Geometry: see drawing. Coordinates: mm, zero at the bounding-box minimum. Give positions to 0.01 mm unless a question says otherwise; leave off trailing zeros. Write each loop counter-clockwise with the first axis right and the second up, starting at its lowest first coordinate (ties: lowest second). Pieces come first, ordered by that corner, then holes. Notation, with made-up numbers: (64, 8.5) - (101, 8.5) arc R20 cw to (101, 21.5) - close; hole circle Ø11 at (26.25, 71). An arc over 180 degrees is marked (long way). Return JSON: item names as keys, results as strings.
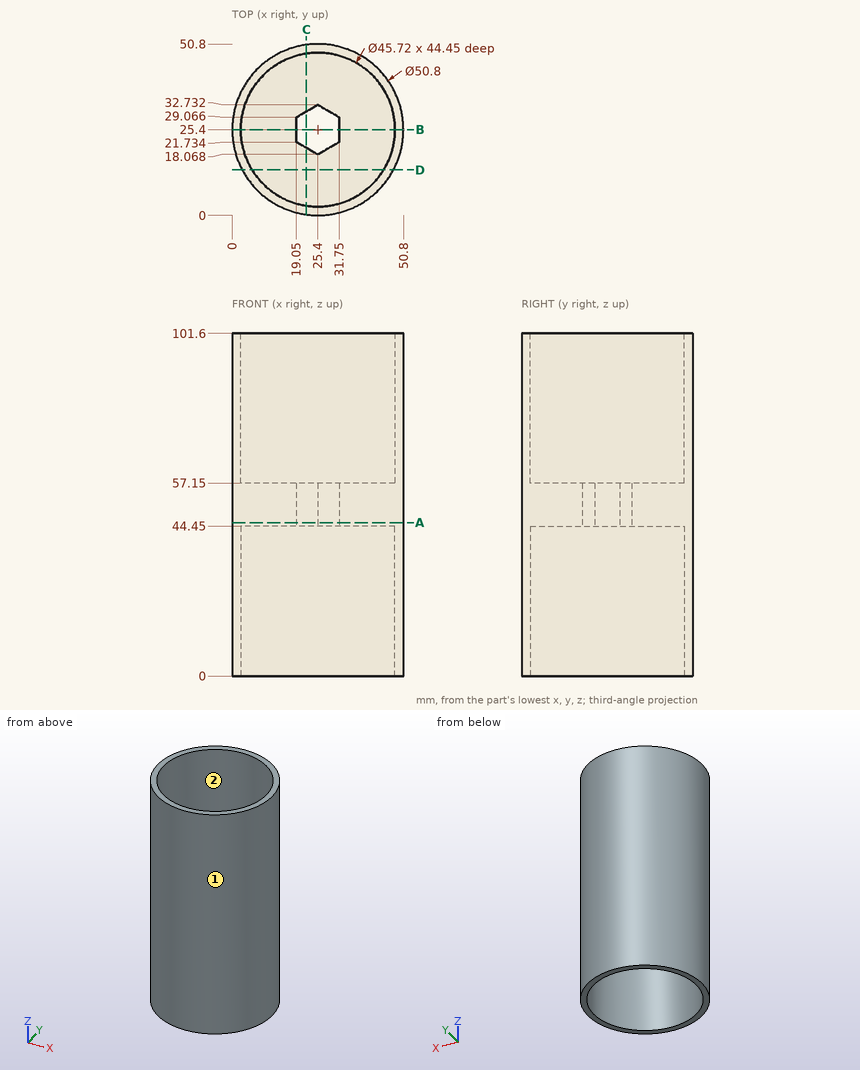
Q1. Mould query, pull axis Y, two halves, no side actions, for the marked faces 1 and 2. Classes: pulls with the +Y half, pulls with the -Y half, needs draft (parallel to the pull), parting line crosses it, or undercut.
Answer key:
{"face 1": "parting line crosses it", "face 2": "undercut"}
Q2. Section query A-A, the plane z = 45.5. Return the cut outline in (x, y).
Answer key:
{"outline": "circle Ø50.8 at (25.4, 25.4); hole (19.05, 21.73) - (25.4, 18.07) - (31.75, 21.73) - (31.75, 29.07) - (25.4, 32.73) - (19.05, 29.07) - close"}
Q3. Section query B-B, the plane y = 25.4. Return the cut outline in (x, z).
Answer key:
{"outline": "(0, 0) - (2.54, 0) - (2.54, 44.45) - (19.05, 44.45) - (19.05, 57.15) - (2.54, 57.15) - (2.54, 101.6) - (0, 101.6) - close; (31.75, 44.45) - (48.26, 44.45) - (48.26, 0) - (50.8, 0) - (50.8, 101.6) - (48.26, 101.6) - (48.26, 57.15) - (31.75, 57.15) - close"}
Q4. Material intervals for probe 1 along Y at (x, z) = (25.4, 12.5); probe 2 along Z at (x, y) = (24.5, 33.5), sorted ascending. Write a range as [from, to].
Answer key:
{"probe 1": "y = [0, 2.54], [48.26, 50.8]", "probe 2": "z = [44.45, 57.15]"}
Q5. Pin query (flat end, axial travel): P1, Ø1.5, axis at x = 18.5, z = 19, coming from the +Y side; P2, Ø4, axis at y = 32.5, z = 16.5, coming from the +X side; P3, Ø6, axis at x = 44, y = 20.5, coming from the +Z side; P4, Ø2, axis at y = 26.5, z = 53, coming from the -X side. Return the tip coordinate at first contact, or that it passes through.
Answer key:
{"P1": "stops at y = 50.04", "P2": "stops at x = 50.28", "P3": "stops at z = 57.15", "P4": "stops at x = 0"}
Q6. Section query C-C, the plane x = 22. Return the cut outline in (y, z), plus the area to 3 significant figures.
Answer key:
{"outline": "(0.23, 0) - (2.79, 0) - (2.79, 44.45) - (20.03, 44.45) - (20.03, 57.15) - (2.79, 57.15) - (2.79, 101.6) - (0.23, 101.6) - close; (30.77, 44.45) - (48.01, 44.45) - (48.01, 0) - (50.57, 0) - (50.57, 101.6) - (48.01, 101.6) - (48.01, 57.15) - (30.77, 57.15) - close", "area": "959 mm^2"}
Q7. Section query D-D, the plane y = 13.5. Return the cut outline in (x, z).
Answer key:
{"outline": "(2.96, 0) - (5.88, 0) - (5.88, 44.45) - (44.92, 44.45) - (44.92, 0) - (47.84, 0) - (47.84, 101.6) - (44.92, 101.6) - (44.92, 57.15) - (5.88, 57.15) - (5.88, 101.6) - (2.96, 101.6) - close"}
